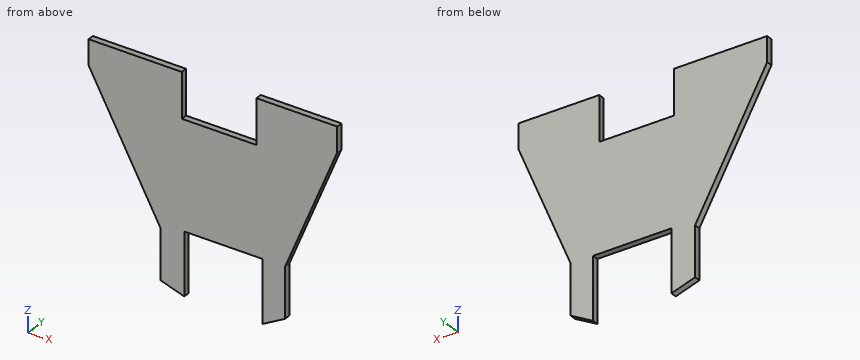
from build123d import *

# Parameters (mm, degrees)
F1_DEPTH = 2.5


# Not quite as in the source:
# - a feature names something its author has since deleted; it is built from what else it names


with BuildPart() as f1:
    # F0 (on Front) → F1 (new body, symmetric)
    with BuildSketch(Plane.XZ):
        Polygon((92, 102), (92, 122), (27, 122), (27, 86), (-33, 86), (-33, 122), (-108, 122), (-108, 102), (-50, -4), (-50, -44), (-31, -50), (-31, 0), (0, 0), (32, 0), (32, -50), (49.9996958359, -40.0000051003), (49.9996958359, -5.1003e-06), align=None)
    extrude(amount=F1_DEPTH, both=True)


solid = f1.part
Build history of the part. All positions in model axes, mm. Give positions to 0.01 mm unless a question says otherwise; leave off trailing zeros. Order: outer loops, then holes, each group sorted by start corner. A loop starts at its lowest first (then second) coordinate and runs counter-clockwise, first axis right, second up. Notation, with made-up numbers: M -3.75,49.5 L 29.25,49.5 A29 ccw 29.25,70.5 Z; hole C 71.5,-10.5 d3. An arc over 180 degrees is marked long. Use one line per item in the form item = value.
1) Saw through at B-B (x = 21). Give the cut face in (y, z).
Calculated:
outline = M -2.5,0 L 2.5,0 L 2.5,86 L -2.5,86 Z
2) Drop flat-ended pins along their axis: pin 1 (1.5 mm diameter, centred on y = 1, z = 99, fed in from -X); pin 2 (1.5 mm diameter, centred on y = -1, z = 3.5, fed in from -X); pin 3 (2.5 mm diameter, centred on y = 0, z = -33.5, fed in from -X). Give the stop position or say it passes through.
Calculated:
pin_1 = -106.77
pin_2 = -54.51
pin_3 = -50
3) Probe probe 1 along X at (y, z) = (-1.55, 108); probe 2 along X at (y, z) = (-1.55, -10.5); probe 3 along Z at (x, y) = (18.5, -0.2). List the from-to ranges inside material, lowest first.
Calculated:
probe_1 = -108 to -33, 27 to 92
probe_2 = -50 to -31, 32 to 50
probe_3 = 0 to 86
4) Saw through at A-A (y = 0). Give the cut face in (x, z), plus the area to 3 significant figures.
Calculated:
outline = M -108,102 L -50,-4 L -50,-44 L -31,-50 L -31,0 L 32,0 L 32,-50 L 50,-40 L 50,0 L 92,102 L 92,122 L 27,122 L 27,86 L -33,86 L -33,122 L -108,122 Z
area = 19,000 mm2
5) Saw through at C-C (z = 73.5). Give the cut face in (x, y).
Calculated:
outline = M -92.41,-2.5 L 80.26,-2.5 L 80.26,2.5 L -92.41,2.5 Z
